```python
from build123d import *

# Parameters (mm, degrees)
PAD_DEPTH    = 9
CHAMFER_SIZE = 1


with BuildPart() as part:
    # Sketch → Pad (new body)
    with BuildSketch(Plane.XY):
        Polygon((18.45, 8.5), (-8.55, 8.5), (-8.55, -8.5), (18.45, -8.5), (18.45, -4.5), (-4.55, -4.5), (-4.55, 4.5), (18.45, 4.5), align=None)
    extrude(amount=PAD_DEPTH)

    # Chamfer
    chamfer_edges = [part.edges().sort_by_distance(p)[0] for p in [
        (18.45, 4.5, 4.5),
        (18.45, -4.5, 4.5),
    ]]
    chamfer(chamfer_edges, length=CHAMFER_SIZE)


solid = part.part
```
CAD build for the part. Positions are in the model's coordinates, mm. A direction names the side the tool comes from. Round coordinates to 2 decimals unless told otherwise and drop trailing zeros. Loops run counter-clockwise (first coordinate to the right, second up) from the corner with the lowest first, then second, coordinate; pieces in that order, holes last. Notation, with made-up numbers: (49, 34) - (99, 34) arc R23 cw to (99, 47) - close; hole circle Ø2 at (18, 68.5). An arc over 180 degrees is marked (long way). Return JSON: item names as keys, results as strings. Group by question number.
Q1. Band-saw the part on C-C on y = 1.25. Give the cut face in (x, z).
Q2. Tool access for faces 1 (the face through (5, 8.5, 4)), 2 (the face through (17.96, 5.01, 4.44)): list every direction of +Z, -Z, +X, -X, +Y, -Y with a clear straight run to the whole face (end or side of a thin tool).
Q3. Flat gauge pins, fed straight in: pin 1 Ø1 at (x, y) = (11.5, 3) entering from -Z; pin 2 Ø4 at (y, z) = (-0.5, 5.5) entering from +X; pin 3 Ø2 at (x, y) = (-4, 4) entering from +Z. Where does each tip first touch, or does it go through?
Q4. Drill centre lines: line 1 along Y through (x, z) = (-2, 7.75); line 2 along X through (y, z) = (-3.75, 0.5). Where is each one in solid material? Low to high. Write a range as [from, to].
Q5. Band-saw the part on A-A on x = 15.5. Give the cut face in (y, z), plus the area to 3 significant figures.
Q6. Two-plate mould, pull along Y, no slides. Class faces 3 (the face through (17.94, -4.99, 4.44)), 4 (the face through (18.45, 7, 4)), 5 (the face through (5, -8.5, 4)): +Y half, -Y half, draft (parallel to the pull), parting line (faces both ways), or undercut.
Q7. Band-saw the part on B-B on z = 1.5. Give the cut face in (x, y).
Solutions:
{
 "1": {"outline": "(-8.55, 0) - (-4.55, 0) - (-4.55, 9) - (-8.55, 9) - close"},
 "2": {"face 1": "+Z, -Z, +X, -X, +Y", "face 2": "+Z, -Z, +X"},
 "3": {"pin 1": "passes through", "pin 2": "stops at x = -4.55", "pin 3": "stops at z = 9"},
 "4": {"line 1": "y = [-8.5, -4.5], [4.5, 8.5]", "line 2": "x = [-8.55, -4.55]"},
 "5": {"outline": "(-8.5, 0) - (-4.5, 0) - (-4.5, 9) - (-8.5, 9) - close; (4.5, 0) - (8.5, 0) - (8.5, 9) - (4.5, 9) - close", "area": "72.0 mm^2"},
 "6": {"face 3": "undercut", "face 4": "draft", "face 5": "-Y half"},
 "7": {"outline": "(-8.55, -8.5) - (18.45, -8.5) - (18.45, -5.5) - (17.45, -4.5) - (-4.55, -4.5) - (-4.55, 4.5) - (17.45, 4.5) - (18.45, 5.5) - (18.45, 8.5) - (-8.55, 8.5) - close"}
}
